Work out the finished part from the listing and answer in its coordinate system (mm). Face numbers are marked on the shaded views. A direction names the side the tool comes from. Give positions to 0.01 mm unless a question says otherwise; leave off trailing zeros. Order: outer loops, then holes, each group sorted by start corner. A loop starts at its lowest first (then second) coordinate and runs counter-clockwise, first axis right, second up. Notation, with made-up numbers: M 62.25,47 L 107.25,47 A33 ccw 107.25,85 Z; hole C 9,88 d7. An arc over 180 degrees is marked long. One line per item, written item: value.
Autodesk Inventor part; units mm, degrees
ref_plane "YZ Plane" through (0, 0, 0) normal (1, 0, 0) x (0, 1, 0)
ref_plane "XZ Plane" through (0, 0, 0) normal (0, 1, 0) x (-1, 0, 0)
ref_plane "XY Plane" through (0, 0, 0) normal (0, 0, 1) x (1, 0, 0)
sketch "Sketch1" plane through (0, 0, 0) normal (0, 1, 0) x (-1, 0, 0)
  line L0 (0, 0) -> (9.5, 0)
  line L1 (9.5, 0) -> (9.5, -64)
  line L2 (9.5, -64) -> (0, -64)
  line L3 (0, -64) -> (0, 0)
  circle A0 centre (3.7, -11.5) radius 2.25
  circle A1 centre (3.7, -59.5) radius 2.25
  line L4 (3.7, -11.5) -> (3.7, -59.5) construction
  dimension "d1" = 9.5
  dimension "d2" = 64
  dimension "d3" = 4.5
  dimension "d4" = 48
  dimension "d6" = 3.7
  dimension "d17" = 4.5
extrude "Extrusion1" add sketch "Sketch1" along normal blind 12
sketch "Sketch2" plane through (-9.5, 0, 0) normal (0, 0, 1) x (1, 0, 0)
  line L0 (9.5, 12) -> (0, 12)
  line L1 (3, 12) -> (8.4, 12)
  line L2 (8.4, 12) -> (8.4, 10.8)
  line L3 (8.4, 10.8) -> (3, 10.8)
  line L4 (3, 10.8) -> (3, 12)
  line L5 (9.5, 0) -> (9.5, 12)
  line L6 (3.55, 0) -> (8.05, 0)
  line L7 (3.55, 12) -> (8.05, 12)
  line L8 (9.5, 0) -> (9.5, 12)
  line L9 (9.5, 0) -> (9.5, 12)
  line L10 (3.55, 12) -> (8.05, 12)
  line L11 (3.55, 12) -> (3.55, 0)
  line L12 (3.55, 12) -> (8.05, 12)
  line L13 (3.55, 0) -> (8.05, 0)
  line L14 (3.55, 12) -> (8.05, 12)
  line L15 (3.55, 0) -> (8.05, 0)
  line L16 (3.55, 12) -> (8.05, 12)
  line L17 (3.55, 0) -> (8.05, 0)
  dimension "d9" = 1.1
  dimension "d10" = 5.4
  dimension "d11" = 1.2
  dimension "d76" = 12
extrude "Extrusion2" cut sketch "Sketch2" against normal up to next
sketch "Sketch3" plane through (0, 0, 0) normal (0, -1, 0) x (1, 0, 0)
  circle A0 centre (-3.7, -11.5) radius 2.25
  circle A1 centre (-3.7, -11.5) radius 3.75
  circle A2 centre (-3.7, -59.5) radius 2.25
  circle A3 centre (-3.7, -59.5) radius 3.75
  point P0 (0, 0)
  dimension "d14" = 7.5
extrude "Extrusion3" cut sketch "Sketch3" against normal blind 3
fillet "Fillet1" radius 1 4 edges at (0, 1.5, -58.8897) (0, 1.5, -60.1103) (0, 1.5, -10.8897) (0, 1.5, -12.1103)
fillet "Fillet2" radius 4 2 edges at (-9.5, 6, -64) (-9.5, 6, 0)
sketch "Sketch28" plane through (0, 0, 0) normal (0, -1, 0) x (1, 0, 0)
  arc A0 (-1.5684, -56.4147) -> (0, -55.592) centre (-1, -55.592) ccw
  line L0 (0, -55.592) -> (0, -53)
  line L1 (0, -15.408) -> (0, -55.592)
  line L2 (-9.5, -60) -> (-9.5, -4)
  line L3 (0, -53) -> (-9.5, -53)
  line L4 (-9.5, -53) -> (-9.5, -31)
  line L5 (-9.5, -31) -> (0, -31)
  line L6 (0, -31) -> (0, -53)
  point P0 (0, 0)
  point P1 (0, -31)
  dimension "d107" = 2.592
  dimension "d108" = 22
extrude "Extrusion19" add sketch "Sketch28" along normal blind 10
sketch "Sketch29" plane through (0, -10, 0) normal (0, -1, 0) x (1, 0, 0)
  line L0 (-9.5, -53) -> (0, -53)
  line L1 (-9.5, -53) -> (38.5, -53)
  line L2 (38.5, -53) -> (38.5, -43)
  line L3 (38.5, -43) -> (-21.5, -43)
  line L4 (-21.5, -43) -> (-21.5, -53)
  line L5 (-21.5, -53) -> (-9.5, -53)
  point P0 (0, 0)
  dimension "d111" = 48
  dimension "d112" = 10
  dimension "d113" = 60
  dimension "d114" = 10
extrude "Extrusion20" add sketch "Sketch29" along normal blind 10
sketch "Sketch32" plane through (0, -20, 0) normal (0, -1, 0) x (1, 0, 0)
  arc A0 (-21.5, -43) -> (38.5, -43) centre (8.5, 103.9694) ccw
  line L0 (-21.5, -43) -> (-21.5, -53)
  line L1 (-21.5, -43) -> (-21.5, -48)
  point P0 (0, 0)
  dimension "d121" = 60
  dimension "d122" = 150
sketch "Sketch34" plane through (0, -20, 0) normal (0, -1, 0) x (1, 0, 0)
  line L0 (-21.5, -43) -> (-21.5, -53)
  line L1 (38.5, -53) -> (38.5, -43)
  arc A0 (-21.5, -48) -> (38.5, -48) centre (8.5, 93.8626) ccw
  point P0 (0, 0)
  dimension "d123" = 145
sketch "Sketch36" plane through (0, -20, 0) normal (0, -1, 0) x (1, 0, 0)
  line L0 (-21.5, -43) -> (-21.5, -53)
  line L1 (-21.5, -48) -> (-21.5, -43)
  line L2 (38.5, -53) -> (38.5, -43)
  line L3 (38.5, -48) -> (38.5, -43)
  point P0 (0, 0)
sketch "Sketch37" plane through (-21.5, -10, -53) normal (-1, 0, 0) x (0, 0, 1)
  arc A0 (10, -10) -> (10, -60) centre (41.225, -35) ccw
  point P0 (53, 10)
  dimension "d126" = 50
  dimension "d127" = 40
properties part number "Back"
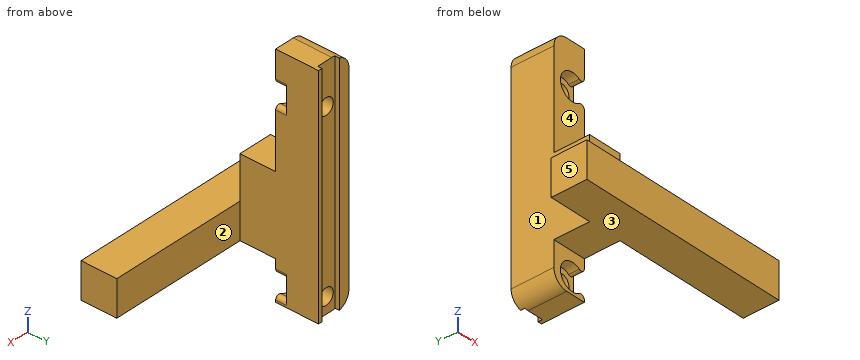
(1) Section A-A, the plane x = -3.7 is taken. Give the vertices of the cut face in (y, z), then the cut area to 3 significant figures.
Findings:
outline: M -20,-53 L 0,-53 L 0,-55.75 L 3,-55.75 L 3,-57.25 L 10.8,-57.25 L 10.8,-13.75 L 3,-13.75 L 3,-15.25 L 0,-15.25 L 0,-31 L -10,-31 L -10,-43 L -20,-43 Z; M 0,-64 L 10.8,-64 L 10.8,-61.75 L 3,-61.75 L 3,-63.25 L 0,-63.25 Z; M 0,-7.75 L 3,-7.75 L 3,-9.25 L 10.8,-9.25 L 10.8,0 L 0,0 Z
area: 896 mm^2
(2) Section C-C, the plane y = 6.5 is taken. Give the vertices of the cut face in (x, z), then the cut area to 3 significant figures.
Findings:
outline: M -9.5,-60 A4 ccw -5.5,-64 L 0,-64 L 0,0 L -5.5,0 A4 ccw -9.5,-4 Z; hole C -3.7,-59.5 d4.5; hole C -3.7,-11.5 d4.5
area: 569 mm^2
(3) Which of the six approach directions +Z, -Z, +X, -X, +Y, -Y give full straight-line access (tool end or side, diameter ignored) to the marked faces 1, 2, 3, 4 and 5?
Findings:
face 1: +Z, -Z, -X, +Y
face 2: +Z, -Z, +X, +Y
face 3: -Z, +X, -X, -Y
face 4: +Z, +X, -X, -Y
face 5: +Z, -Z, -X, +Y, -Y
(4) Find the intervals of material crossed by probe 1 along Z at (x, y) = (-3.7, 8.5); probe 2 along Z at (x, y) = (-3.7, 2.1); probe 3 along X at (y, z) = (8.25, -59.5), in increasing order. Write a range as from..to.
Findings:
probe 1: z = -64..-61.75, -57.25..-13.75, -9.25..0
probe 2: z = -64..-63.25, -55.75..-15.25, -7.75..0
probe 3: x = -9.5..-5.95, -1.45..0
(5) Given P1, Ø1, axis at y = 11.5, z = -23.5, coming from the +X side; P2, Ø1.3, axis at y = 11.5, z = -23.5, coming from the -X side; P3, Ø3, axis at x = -2, y = -16, coming from the +Z side, each flat-ended and moving along its own axis, determine where each tip first touches the part or whether it passes through.
Findings:
P1: stops at x = 0
P2: stops at x = -9.5
P3: stops at z = -43
(6) Section D-D, the plane z = -47.5 is taken. Give the vertices of the cut face in (x, y), then the cut area to 3 significant figures.
Findings:
outline: M -21.5,-20 L 38.5,-20 L 38.5,-10 L 0,-10 L 0,12 L -1.1,12 L -1.1,10.8 L -6.5,10.8 L -6.5,12 L -9.5,12 L -9.5,-10 L -21.5,-10 Z
area: 803 mm^2
(7) Section B-B, the plane z = -11.5 is taken. Give the vertices of the cut face in (x, y).
Findings:
outline: M -9.5,0 L -7.45,0 L -7.45,3 L -5.95,3 L -5.95,10.8 L -6.5,10.8 L -6.5,12 L -9.5,12 Z; M -1.45,3 L 0,3 L 0,12 L -1.1,12 L -1.1,10.8 L -1.45,10.8 Z
